Work out the finished part from the listing and answer in its coordinate system (mm). Face numbers are marked on the shaded views. Coordinates: 2 decimals unless noted, no trailing zeros. Order: outer loops, then holes, each group sorted by start corner. A loop starts at its lowest first (then second) coordinate and runs counter-clockwise, first axis right, second up. Notation, with made-up numbers: M 89.5,13 L 144.5,13 A31 cw 144.5,42 Z; hole C 2.5,58.5 d11. An arc over 180 degrees is marked long. Use a Markdown table: item, result.
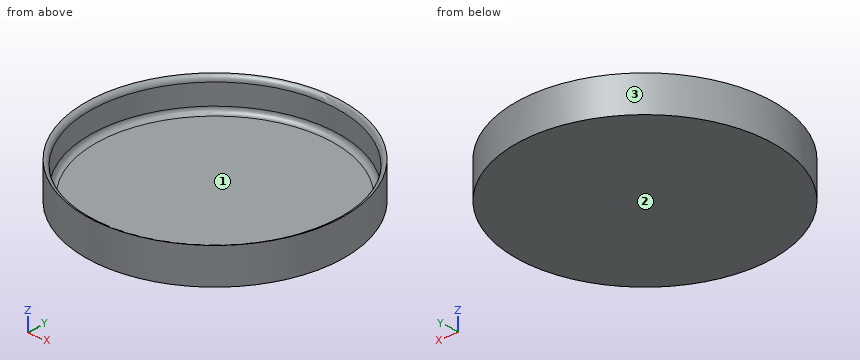
from build123d import *

# Parameters (mm, degrees)
F0_R     = 71.2988650601
F1_DEPTH = 20
F2_T     = -2.5
F3_R     = 3


# Not quite as in the source:
# - a fillet or chamfer that OpenCascade refuses, or shapes differently, is made with other operations: its cross-section is extruded or revolved along the edge and cut away or added


with BuildPart() as f1:
    # F0 (on Top) → F1 (new body)
    with BuildSketch(Plane.XY):
        Circle(F0_R)
    extrude(amount=F1_DEPTH)

    # F2
    f2_openings = [f1.faces().sort_by_distance(p)[0] for p in [
        (0, 0, 20),
    ]]
    offset(amount=F2_T, openings=f2_openings)

    # F3
    f3_edges = [f1.edges().sort_by_distance(p)[0] for p in [
        (-68.798865, 0, 2.5),
    ]]
    fillet(f3_edges, radius=F3_R)

    # F4: fillet of radius 3 on 1 edges, made by hand

    # F4_s1 → F4_t2 (revolve, cut)
    with BuildSketch(Plane.XZ):
        with BuildLine():
            ThreePointArc((68.7988650601, 17.0419601084), (69.5075772126, 18.9784517816), (71.2988650601, 20))
            Line((71.2988650601, 20), (68.7988650601, 20))
            Line((68.7988650601, 20), (68.7988650601, 17.0419601084))
        make_face()
    revolve(axis=Axis((0, 0, 20), (0, 0, 1)), mode=Mode.SUBTRACT)


solid = f1.part
1. Section A-A on y = 0 is taken. Determine the outline of the cut face in (x, z), then the cut area to 3 significant figures.
Answers below:
| item | result |
|---|---|
| outline | M -71.3,0 L 71.3,0 L 71.3,20 A3 ccw 68.8,17.04 L 68.8,5.5 A3 cw 65.8,2.5 L -65.8,2.5 A3 cw -68.8,5.5 L -68.8,17.04 A3 ccw -71.3,20 Z |
| area | 444 mm² |
2. Find the intervals of material crossed by probe 1 along Y at (x, z) = (2, 13); probe 2 along Z at (x, y) = (15, -25); probe 3 along X at (y, z) = (-28, 17), in increasing order.
Answers below:
| item | result |
|---|---|
| probe 1 | -71.27 to -68.77, 68.77 to 71.27 |
| probe 2 | 0 to 2.5 |
| probe 3 | -65.57 to -62.84, 62.84 to 65.57 |
3. For a pull along Y with two mould halves and no side action, classify the marked faces 1, 2 and 3 as +Y half, -Y half, draft (parallel to the pull), parting line (faces both ways), or undercut.
Answers below:
| item | result |
|---|---|
| face 1 | undercut |
| face 2 | draft |
| face 3 | parting line |
4. Section C-C on z = 10 is taken. Determine the outline of the cut face in (x, y).
Answers below:
| item | result |
|---|---|
| outline | C 0,0 d142.6; hole C 0,0 d137.6 |
5. Flat-ended cylindrical pins translate along their axes: P1, Ø1, axis at x = -48.5, z = 6, coming from the +Y side; P2, Ø6, axis at y = -54, z = 14, coming from the +X side (3 decimals); P3, Ø2, axis at x = 23.5, z = 11, coming from the -Y side; P4, Ø6, axis at x = 31, y = -34, coming from the -Z side. Find the tip coordinate at first contact, or state that the pin passes through.
Answers below:
| item | result |
|---|---|
| P1 | y = 52.72 |
| P2 | x = 49.825 |
| P3 | y = -67.66 |
| P4 | z = 0 |
